from build123d import *

# Parameters (mm, degrees)
EXTRUDE_1_DEPTH     = 2
SKETCH_2_W          = 6
SKETCH_2_H          = 35
EXTRUDE_2_DEPTH     = 60
FILLET_1_R          = 17.5
SKETCH_3_R          = 16
CUT_EXTRUDE_1_DEPTH = 5
CHAMFER_1_SIZE      = 1.640243073
CHAMFER_1_SIZE_2    = 0.8
SKETCH_4_R          = 15
CUT_EXTRUDE_2_DEPTH = 102.631713982
SKETCH_5_W          = 25
SKETCH_5_H          = 10.5
EXTRUDE_3_DEPTH     = 7.3
EXTRUDE_4_DEPTH     = 2
FILLET_2_R          = 1
EXTRUDE_5_DEPTH     = 5
SKETCH_9_R          = 1.15
CUT_EXTRUDE_3_DEPTH = 98.627174941
SKETCH_10_R         = 2
CUT_EXTRUDE_4_DEPTH = 10
FILLET_3_R          = 0.5


# Some blends are built 0.0001 mm under size
with BuildPart() as part:
    # 스케치1 → 보스-돌출1 (new body)
    with BuildSketch(Plane(origin=(0, 0, 0), x_dir=(1, 0, 0), z_dir=(0, 1, 0))):
        with BuildLine():
            Line((-11.151844037, -1.536211432), (-64.981844037, -1.536211432))
            ThreePointArc((-64.981844037, -1.536211432), (-49.250859027, -42.418779863), (-11.151844037, -64.036211432))
            Line((-11.151844037, -64.036211432), (-11.151844037, -1.536211432))
        make_face()
    extrude(amount=EXTRUDE_1_DEPTH)

    # 스케치2 → 보스-돌출2 (add)
    with BuildSketch(Plane(origin=(0, 2, 0), x_dir=(1, 0, 0), z_dir=(0, 1, 0))):
        with Locations((-14.151844037, -19.036211432)):
            Rectangle(SKETCH_2_W, SKETCH_2_H)
    extrude(amount=EXTRUDE_2_DEPTH)

    # 필렛1
    fillet_1_edges = [part.edges().sort_by_distance(p)[0] for p in [
        (-14.151844037, 62, 1.536211432),
        (-14.151844037, 62, 36.536211432),
    ]]
    fillet(fillet_1_edges, radius=FILLET_1_R - 0.0001)  # a hair under: the kernel refuses the full size

    # 스케치3 → 컷-돌출1 (cut)
    with BuildSketch(Plane(origin=(-11.151844037, 0, 0), x_dir=(0, 0, -1), z_dir=(1, 0, 0))):
        with Locations((-19.036211432, 44.5)):
            Circle(SKETCH_3_R)
    extrude(amount=-CUT_EXTRUDE_1_DEPTH, mode=Mode.SUBTRACT)

    # 모따기1
    # the kernel refuses this chamfer: 1.640243073, 0.8 mm, written as the material it takes off along each edge
    with BuildSketch(Plane(origin=(-11.151844037, 44.5, 19.036211432), x_dir=(0, 0, -1), z_dir=(0, -1, 0))) as chamfer_1_piece_1:
        Polygon((16 + CHAMFER_1_SIZE, 0), (16, -CHAMFER_1_SIZE_2), (16, 0), align=None)
    revolve(axis=Axis((-11.151844037, 44.5, 19.036211432), (1, 0, 0)), mode=Mode.SUBTRACT)

    # 스케치4 → 컷-돌출2 (cut, through all)
    with BuildSketch(Plane(origin=(-16.151844037, 0, 0), x_dir=(0, 0, -1), z_dir=(1, 0, 0))):
        with Locations((-19.036211432, 44.5)):
            Circle(SKETCH_4_R)
    extrude(amount=-CUT_EXTRUDE_2_DEPTH, mode=Mode.SUBTRACT)

    # 스케치5 → 보스-돌출3 (add)
    with BuildSketch(Plane(origin=(0, 2, 0), x_dir=(1, 0, 0), z_dir=(0, 1, 0))):
        with Locations((-32.651844037, -6.786211432)):
            Rectangle(SKETCH_5_W, SKETCH_5_H)
        with Locations((-32.651844037, -31.286211432)):
            Rectangle(SKETCH_5_W, SKETCH_5_H)
    extrude(amount=EXTRUDE_3_DEPTH)

    # 스케치6 → 보스-돌출4 (add)
    with BuildSketch(Plane(origin=(0, 9.3, 0), x_dir=(1, 0, 0), z_dir=(0, 1, 0))):
        Polygon((-45.151844037, -31.536211432), (-25.151844037, -31.536211432), (-25.151844037, -26.036211432), (-20.151844037, -26.036211432), (-20.151844037, -36.536211432), (-45.151844037, -36.536211432), align=None)
        Polygon((-45.151844037, -1.536211432), (-20.151844037, -1.536211432), (-20.151844037, -12.036211432), (-25.151844037, -12.036211432), (-25.151844037, -6.536211432), (-45.151844037, -6.536211432), align=None)
    extrude(amount=EXTRUDE_4_DEPTH)

    # 필렛2
    fillet_2_edges = [part.edges().sort_by_distance(p)[0] for p in [
        (-45.151844037, 6.65, 1.536211432),
        (-45.151844037, 5.65, 12.036211432),
        (-45.151844037, 5.65, 26.036211432),
        (-45.151844037, 6.65, 36.536211432),
    ]]
    fillet(fillet_2_edges, radius=FILLET_2_R)

    # 스케치7 → 보스-돌출5 (add)
    with BuildSketch(Plane.ZY.offset(25.151844037)):
        with BuildLine():
            Line((1.536211432, 11.3), (12.036211432, 11.3))
            Line((12.036211432, 11.3), (12.036211432, 36.014718626))
            ThreePointArc((12.036211432, 36.014718626), (9.884247068, 38.397414624), (8.511953739, 41.3))
            Line((8.511953739, 41.3), (1.536211432, 41.3))
            Line((1.536211432, 41.3), (1.536211432, 11.3))
        make_face()
        with BuildLine():
            Line((36.536211432, 11.3), (26.036211432, 11.3))
            Line((26.036211432, 11.3), (26.036211432, 36.014718626))
            ThreePointArc((26.036211432, 36.014718626), (28.188175797, 38.397414624), (29.560469126, 41.3))
            Line((29.560469126, 41.3), (36.536211432, 41.3))
            Line((36.536211432, 41.3), (36.536211432, 11.3))
        make_face()
    extrude(amount=-EXTRUDE_5_DEPTH)

    # 스케치9 → 컷-돌출3 (cut, through all)
    with BuildSketch(Plane.ZY.offset(25.151844037)):
        with Locations((8.786211432, 35.8)):
            Circle(SKETCH_9_R)
        with Locations((8.786211432, 15.3)):
            Circle(SKETCH_9_R)
        with Locations((29.286211432, 15.3)):
            Circle(SKETCH_9_R)
        with Locations((29.286211432, 35.8)):
            Circle(SKETCH_9_R)
    extrude(amount=-CUT_EXTRUDE_3_DEPTH, mode=Mode.SUBTRACT)

    # 스케치10 → 컷-돌출4 (cut)
    with BuildSketch(Plane(origin=(-11.151844037, 0, 0), x_dir=(0, 0, -1), z_dir=(1, 0, 0))):
        with Locations((-29.286211432, 15.3)):
            Circle(SKETCH_10_R)
        with Locations((-8.786211432, 15.3)):
            Circle(SKETCH_10_R)
        with Locations((-8.786211432, 35.8)):
            Circle(SKETCH_10_R)
        with Locations((-29.286211432, 35.8)):
            Circle(SKETCH_10_R)
    extrude(amount=-CUT_EXTRUDE_4_DEPTH, mode=Mode.SUBTRACT)

    # 필렛3
    fillet_3_edges = [part.edges().sort_by_distance(p)[0] for p in [
        (-45.151844037, 10.3, 31.536211432),
        (-25.151844037, 22.657359313, 26.036211432),
        (-35.151844037, 9.3, 31.536211432),
        (-45.151844037, 9.3, 29.286211432),
        (-44.858950818, 9.3, 26.329104651),
        (-34.651844037, 9.3, 12.036211432),
        (-44.858950818, 9.3, 11.743318213),
        (-45.151844037, 9.3, 8.786211432),
        (-35.151844037, 9.3, 6.536211432),
        (-45.151844037, 10.3, 6.536211432),
        (-25.151844037, 22.657359313, 12.036211432),
        (-34.651844037, 9.3, 26.036211432),
    ]]
    fillet(fillet_3_edges, radius=FILLET_3_R)


solid = part.part
Can you work these out from the model? Positions are in its coordinate system, mm. A direction names the side the tool comes from. Give positions to 0.01 mm unless a question says otherwise; leave off trailing zeros. Loops run counter-clockwise (first coordinate to the right, second up) from the corner with the lowest first, then second, coordinate; pieces in that order, holes last. Notation, with made-up numbers: M 24.5,74 L 48.5,74 A10 cw 48.5,88 Z; hole C 33,-17.75 d3. An arc over 180 degrees is marked long. One line per item, written item: value. Start each with the question number.
1) I'm going to push flat-ended pins straight in: pin 1 (5.5 mm diameter, centred on x = -36.5, z = 5.5, fed in from +Y); pin 2 (2 mm diameter, centred on y = 39, z = 32, fed in from -X); pin 3 (1.5 mm diameter, centred on x = -19.5, z = 46, fed in from +Y). Where does each tip first touch, or does it pass through?
2) If we section it at D-D, the plane z = 38.5: Write out the boundary of the cut face in (x, y), and give its area (3 significant figures).
3) Thinking about a two-plate mould opening in Y: for faces 1 (the face through (-23.18, 36.94, 29.14)), 2 (the face through (-14, 23, 36.536)), 3 (the face through (-23.18, 36.94, 8.64)), 4 (the face through (-22.69, 38.36, 9.91)), which applies, +Y half, -Y half, draft (parallel to the pull), parting line (faces both ways), or undercut?
4) If we section it at A-A, the plane y = 18.5: Write out the boundary of the cut face in (x, z), and give its area (3 significant figures).
5) If we section it at B-B, the plane x = -39: Write out the boundary of the cut face in (y, z).
6) If we section it at C-C, the plane x = -27.5: Write out the boundary of the cut face in (y, z).
7) On a 3-axis mill with a long thin cutter (end or side, diameter ignored), from which of +Z, -Z, +X, -X, +Y, -Y can I reach the whole of each face in a straight line? I mean faces 5 (the face through (-14.02, 55.31, 30.83)), 6 (the face through (-17.152, 25, 19)), 7 (the face through (-45.152, 7, 7)). Say none if no direction works.
8) If I drill on line 1 (Y direction, x = -13.5, z = 19); line 2 (X direction, y = 29, z = 9); line 3 (Y direction, x = -23, z = 38), over which ranges is the centre line in solid material (lowest first)? Write a range as [from, to].
Completed:
1. pin 1: stops at y = 11.3
1. pin 2: stops at x = -25.15
1. pin 3: stops at y = 2
2. outline: M -52.37,0 L -11.15,0 L -11.15,2 L -52.37,2 Z
2. area: 82.4 mm^2
3. face 1: undercut
3. face 2: draft
3. face 3: undercut
3. face 4: +Y half
4. outline: M -25.15,1.54 L -20.15,1.54 L -20.15,12.04 L -24.65,12.04 A0.5 ccw -25.15,11.54 Z; M -25.15,26.54 A0.5 ccw -24.65,26.04 L -20.15,26.04 L -20.15,36.54 L -25.15,36.54 Z; M -17.15,1.54 L -11.15,1.54 L -11.15,36.54 L -17.15,36.54 Z
4. area: 315 mm^2
5. outline: M 0,1.54 L 11.3,1.54 L 11.3,6.54 L 9.8,6.54 A0.5 cw 9.3,7.04 L 9.3,11.54 A0.5 ccw 8.8,12.04 L 2,12.04 L 2,26.04 L 8.8,26.04 A0.5 ccw 9.3,26.54 L 9.3,31.04 A0.5 cw 9.8,31.54 L 11.3,31.54 L 11.3,36.54 L 2,36.54 L 2,52 L 0,52 Z
6. outline: M 0,1.54 L 11.3,1.54 L 11.3,6.54 L 9.8,6.54 A0.5 cw 9.3,7.04 L 9.3,11.54 A0.5 ccw 8.8,12.04 L 2,12.04 L 2,26.04 L 8.8,26.04 A0.5 ccw 9.3,26.54 L 9.3,31.04 A0.5 cw 9.8,31.54 L 11.3,31.54 L 11.3,36.54 L 2,36.54 L 2,58.9 L 0,58.9 Z
7. face 5: +X
7. face 6: +Z, -Z, +Y
7. face 7: +Z, -Z, -X, +Y
8. line 1: y = [0, 28.5], [60.5, 62]
8. line 2: x = [-25.15, -20.15], [-17.15, -11.15]
8. line 3: y = [0, 2]
